Geometry: final body of the model. Coordinates: model frame, mm. Give positions to 0.01 mm unless a question says otherwise; leave off trailing zeros. Write each loop counter-clockwise with the first axis right and the second up, starting at its lowest first coordinate (ties: lowest second). Pieces come first, ordered by that corner, then holes. Notation, with made-up numbers: (10.5, 5.5) -> (38.5, 5.5) arc R25 cw to (38.5, 27.5) -> close; hole circle Ø7 at (4.5, 8.25). An arc over 180 degrees is marked (long way). Answer in a Markdown table with one row per item. Add a question column.
Item 1: First-contact query: P1, Ø0.5, axis at y = -0.5, z = 136, coming from the -X side; P2, Ø0.5, axis at x = 236, y = -0.5, coming from the -Z side; P3, Ø0.5, axis at x = 271.5, y = -0.5, coming from the -Z side; P4, Ø4, axis at x = 109.45, z = 133.35, coming from the -Y side. Flat tips, straight axial feed; report the tip coordinate or a pass-through.
Item 2: Section query A-A on y = -0.85. State how many separate pieces and enclosed holes the cut face has, plus the area to 3 significant figures.
Item 3: Section query B-B on x = -126. Output: boundary loops of the cut face in (y, z), plus the area to 3 significant figures.
Item 4: Material intervals for probe 1 along X at (y, z) = (-0.15, 133.35); probe 2 along X at (y, z) = (-0.5, -246.5); probe 3 along Z at (x, y) = (33.5, -0.65), sorted ascending. Write a range as from..to.
Item 5: Section query C-C on z = -204. Output: boundary loops of the cut face in (x, y).
```python
from build123d import *

# Parameters (mm, degrees)
SKETCH1_W          = 609.6
SKETCH1_H          = 254
BASE_FLANGE1_DEPTH = 1
SKETCH6_W          = 25.4
SKETCH6_H          = 25.4
TAB2_DEPTH         = 1
SKETCH11_W         = 25.4
SKETCH11_H         = 25.4
TAB3_DEPTH         = 1
SKETCH14_W         = 203.2
SKETCH14_H         = 203.2
TAB4_DEPTH         = 1
SKETCH17_W         = 127
SKETCH17_H         = 12.7
TAB5_DEPTH         = 1
SKETCH20_W         = 127
SKETCH20_H         = 12.7
TAB7_DEPTH         = 1
SKETCH25_W         = 12.7
SKETCH25_H         = 12.7
TAB8_DEPTH         = 1
SKETCH28_W         = 12.7
SKETCH28_H         = 12.7
TAB10_DEPTH        = 1
SKETCH36_R         = 3.15
CUT_EXTRUDE2_DEPTH = 450.372985392
SKETCH38_R         = 3.15
CUT_EXTRUDE3_DEPTH = 450.372985392


# Sheet-metal steps are written as plain solids
with BuildPart() as part:
    # Sketch1 → Base-Flange1 (new body)
    with BuildSketch(Plane(origin=(0, 0, 0), x_dir=(1, 0, 0), z_dir=(0, 1, 0))):
        Rectangle(SKETCH1_W, SKETCH1_H)
    extrude(amount=-BASE_FLANGE1_DEPTH)

    # Sketch6 → Tab2 (add)
    with BuildSketch(Plane(origin=(0, 0, 0), x_dir=(1, 0, 0), z_dir=(0, 1, 0))):
        with Locations((-241.3, 139.7)):
            Rectangle(SKETCH6_W, SKETCH6_H)
    extrude(amount=-TAB2_DEPTH)

    # Sketch11 → Tab3 (add)
    with BuildSketch(Plane(origin=(0, 0, 0), x_dir=(1, 0, 0), z_dir=(0, 1, 0))):
        with Locations((241.3, 139.7)):
            Rectangle(SKETCH11_W, SKETCH11_H)
    extrude(amount=-TAB3_DEPTH)

    # Sketch14 → Tab4 (add)
    with BuildSketch(Plane(origin=(0, 0, 0), x_dir=(1, 0, 0), z_dir=(0, 1, 0))):
        with Locations((0, 228.6)):
            Rectangle(SKETCH14_W, SKETCH14_H)
    extrude(amount=-TAB4_DEPTH)

    # Sketch17 → Tab5 (add)
    with BuildSketch(Plane(origin=(0, 0, 0), x_dir=(1, 0, 0), z_dir=(0, 1, 0))):
        with Locations((-213.36, -133.35)):
            Rectangle(SKETCH17_W, SKETCH17_H)
    extrude(amount=-TAB5_DEPTH)

    # Sketch20 → Tab7 (add)
    with BuildSketch(Plane(origin=(0, 0, 0), x_dir=(1, 0, 0), z_dir=(0, 1, 0))):
        with Locations((213.36, -133.35)):
            Rectangle(SKETCH20_W, SKETCH20_H)
    extrude(amount=-TAB7_DEPTH)

    # Sketch25 → Tab8 (add)
    with BuildSketch(Plane(origin=(0, 0, 0), x_dir=(1, 0, 0), z_dir=(0, 1, 0))):
        with Locations((-109.45, -133.35)):
            Rectangle(SKETCH25_W, SKETCH25_H)
    extrude(amount=-TAB8_DEPTH)

    # Sketch28 → Tab10 (add)
    with BuildSketch(Plane(origin=(0, 0, 0), x_dir=(1, 0, 0), z_dir=(0, 1, 0))):
        with Locations((109.45, -133.35)):
            Rectangle(SKETCH28_W, SKETCH28_H)
    extrude(amount=-TAB10_DEPTH)

    # Sketch36 → Cut-Extrude2 (cut, through all)
    with BuildSketch(Plane(origin=(0, 0, 0), x_dir=(1, 0, 0), z_dir=(0, 1, 0))):
        with Locations(Location((-109.45, -133.35, 0), (0, 0, 270))):
            Circle(SKETCH36_R)
    extrude(amount=-CUT_EXTRUDE2_DEPTH, mode=Mode.SUBTRACT)

    # Sketch38 → Cut-Extrude3 (cut, through all)
    with BuildSketch(Plane(origin=(0, 0, 0), x_dir=(1, 0, 0), z_dir=(0, 1, 0))):
        with Locations(Location((109.45, -133.35, 0), (0, 0, 270))):
            Circle(SKETCH38_R)
    extrude(amount=-CUT_EXTRUDE3_DEPTH, mode=Mode.SUBTRACT)


solid = part.part
```
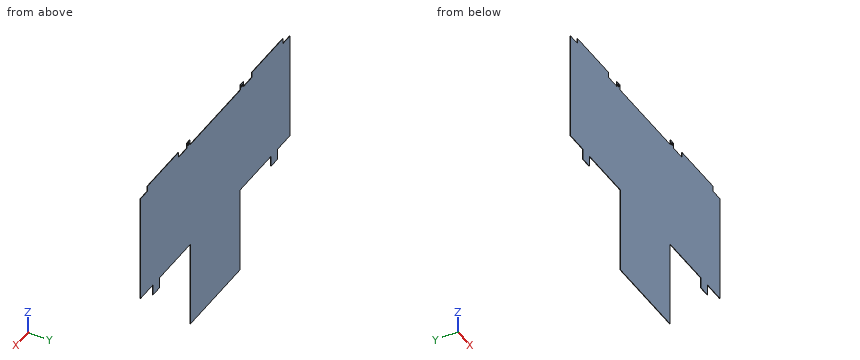
Findings below:
| question | item | result |
|---|---|---|
| 1 | P1 | stops at x = -276.86 |
| 1 | P2 | stops at z = -152.4 |
| 1 | P3 | stops at z = -127 |
| 1 | P4 | passes through |
| 2 | separate pieces | 1 |
| 2 | enclosed holes | 2 |
| 2 | area | 201,000 mm^2 |
| 3 | outline | (-1, -127) -> (0, -127) -> (0, 127) -> (-1, 127) -> close |
| 3 | area | 254 mm^2 |
| 4 | probe 1 | x = -276.86..-149.86, -115.8..-112.6, -106.3..-103.1, 103.1..106.3, 112.6..115.8, 149.86..276.86 |
| 4 | probe 2 | x = -101.6..101.6 |
| 4 | probe 3 | z = -330.2..127 |
| 5 | outline | (-101.6, -1) -> (101.6, -1) -> (101.6, 0) -> (-101.6, 0) -> close |
